from build123d import *

# Parameters (mm, degrees)
SKETCH1_W           = 30
SKETCH1_H           = 15
BOSS_EXTRUDE1_DEPTH = 2
SKETCH2_W           = 6.5
SKETCH2_H           = 15
BOSS_EXTRUDE2_DEPTH = 4
SKETCH3_W           = 6.5
SKETCH3_H           = 2
BOSS_EXTRUDE3_DEPTH = 10
SKETCH4_R           = 2
CUT_EXTRUDE2_DEPTH  = 5
BOSS_EXTRUDE4_START = 5
SKETCH5_R           = 3.5
SKETCH5_R_2         = 2
BOSS_EXTRUDE4_DEPTH = 5


with BuildPart() as part:
    # Sketch1 → Boss-Extrude1 (new body)
    with BuildSketch(Plane(origin=(0, 0, 0), x_dir=(0, 0, -1), z_dir=(1, 0, 0))):
        with Locations((15, 7.5)):
            Rectangle(SKETCH1_W, SKETCH1_H)
    extrude(amount=BOSS_EXTRUDE1_DEPTH)

    # Sketch2 → Boss-Extrude2 (add)
    with BuildSketch(Plane(origin=(0, 0, -30), x_dir=(-1, 0, 0), z_dir=(0, 0, -1))):
        with Locations((-3.25, 7.5)):
            Rectangle(SKETCH2_W, SKETCH2_H)
    extrude(amount=BOSS_EXTRUDE2_DEPTH)

    # Sketch3 → Boss-Extrude3 (add)
    with BuildSketch(Plane(origin=(0, 0, -34), x_dir=(-1, 0, 0), z_dir=(0, 0, -1))):
        with Locations((-3.25, 7.5)):
            Rectangle(SKETCH3_W, SKETCH3_H)
    extrude(amount=BOSS_EXTRUDE3_DEPTH)

    # Sketch4 → Cut-Extrude2 (cut)
    with BuildSketch(Plane(origin=(2, 0, 0), x_dir=(0, 0, -1), z_dir=(1, 0, 0))):
        with Locations((10, 7.5)):
            Circle(SKETCH4_R)
    extrude(amount=-CUT_EXTRUDE2_DEPTH, mode=Mode.SUBTRACT)

    # Sketch5 → Boss-Extrude4 (add)
    with BuildSketch(Plane(origin=(2, 0, 0), x_dir=(0, 0, -1), z_dir=(1, 0, 0)).offset(BOSS_EXTRUDE4_START)):
        with Locations(Location((10, 7.5, 0), (0, 0, 180))):
            Circle(SKETCH5_R)
        with Locations((10, 7.5)):
            Circle(SKETCH5_R_2, mode=Mode.SUBTRACT)
    extrude(amount=-BOSS_EXTRUDE4_DEPTH)


solid = part.part
Source: CAD feature listing. Evaluate the final solid. Frame: model axes, mm. A direction names the side the tool comes from. Round coordinates to 2 decimals unless told otherwise and drop trailing zeros. Loops run counter-clockwise (first coordinate to the right, second up) from the corner with the lowest first, then second, coordinate; pieces in that order, holes last. Notation, with made-up numbers: (83, 38.5) - (131, 38.5) arc R32 ccw to (131, 76.5) - close; hole circle Ø11 at (4.5, -36.5). An arc over 180 degrees is marked (long way). Write item = value, one per line. Start each with the question number.
Item 1: Reachability of faces 4 (the face through (6.5, 7, -34)), 5 (the face through (4, 8, -30)), 6 (the face through (3, 3, -34)), 7 (the face through (3, 8.5, -39)) from +Z, -Z, +X, -X, +Y, -Y: full face, straight path, thin tool, end or side. Return the list, or none.
Item 2: Mould query, pull axis Y, two halves, no side actions, for faces 1 (the face through (3.549, 9.483, -9.74)), 2 (the face through (1, 0, -21)), 3 (the face through (4.5, 9.6, -12.8)). Classes: released by +Y, released by -Y, zero draft, split by the parting line, or undercut.
Item 3: Section query C-C on y = 7.5. Output: boundary loops of the cut face in (x, z).
Item 4: Section query B-B on z = -10. Output: boundary loops of the cut face in (x, y), plus the area to 3 significant figures.
Item 5: Material intervals for line 1 (Y direction, x = 2.5, z = -10); line 2 (Z direction, x = 5, y = 8.25); line 3 (Z direction, x = 1.5, y = 12), sorted ascending.
Item 6: Section query A-A on x = 5.25. Output: boundary loops of the cut face in (y, z).
Item 7: Section query D-D on x = 0.5. Output: boundary loops of the cut face in (y, z), plus the area to 3 significant figures.
Item 8: First-contact query: pin 1 Ø4 at (x, y) = (6.5, 3.5) entering from +Z; pin 2 Ø2 at (x, z) = (3, -39) entering from +Y; pin 3 Ø2 at (x, y) = (3, 13) entering from -Z; pin 4 Ø4 at (x, z) = (1.5, -10) entering from -Y. Flat tips, straight axial feed; report the tip coordinate or a pass-through.
Results list:
q1.face_4 = -Z, +X, +Y, -Y
q1.face_5 = +X, +Y, -Y
q1.face_6 = -Z, +X, -X, -Y
q1.face_7 = -Z, +X, -X, +Y
q2.face_1 = undercut
q2.face_2 = released by -Y
q2.face_3 = split by the parting line
q3.outline = (0, -44) - (6.5, -44) - (6.5, -30) - (2, -30) - (2, -13.5) - (7, -13.5) - (7, -12) - (0, -12) - close; (0, -8) - (7, -8) - (7, -6.5) - (2, -6.5) - (2, 0) - (0, 0) - close
q4.outline = (0, 0) - (2, 0) - (2, 4) - (7, 4) - (7, 5.5) - (0, 5.5) - close; (0, 9.5) - (7, 9.5) - (7, 11) - (2, 11) - (2, 15) - (0, 15) - close
q4.area = 37.0 mm²
q5.line_1 = 4 to 5.5, 9.5 to 11
q5.line_2 = -44 to -30, -13.42 to -11.85, -8.15 to -6.58
q5.line_3 = -34 to 0
q6.outline = (0, -34) - (6.5, -34) - (6.5, -44) - (8.5, -44) - (8.5, -34) - (15, -34) - (15, -30) - (0, -30) - close; circle Ø7 at (7.5, -10); hole circle Ø4 at (7.5, -10)
q7.outline = (0, -34) - (6.5, -34) - (6.5, -44) - (8.5, -44) - (8.5, -34) - (15, -34) - (15, 0) - (0, 0) - close; hole circle Ø4 at (7.5, -10)
q7.area = 517 mm²
q8.pin_1 = -7.13
q8.pin_2 = 8.5
q8.pin_3 = -34
q8.pin_4 = 0
